Verification items for the finished model (mm, model axes). Face numbers are marked on the shaded views. A direction names the side the tool comes from. Round coordinates to 2 decimals unless told otherwise and drop trailing zeros. Order: outer loops, then holes, each group sorted by start corner. A loop starts at its lowest first (then second) coordinate and runs counter-clockwise, first axis right, second up. Notation, with made-up numbers: M 66.5,11 L 71.5,11 A16 ccw 71.5,18 Z; hole C 52.5,8 d11. An arc over 180 degrees is marked long. Return JSON: item names as keys, results as strings. Group by question number.
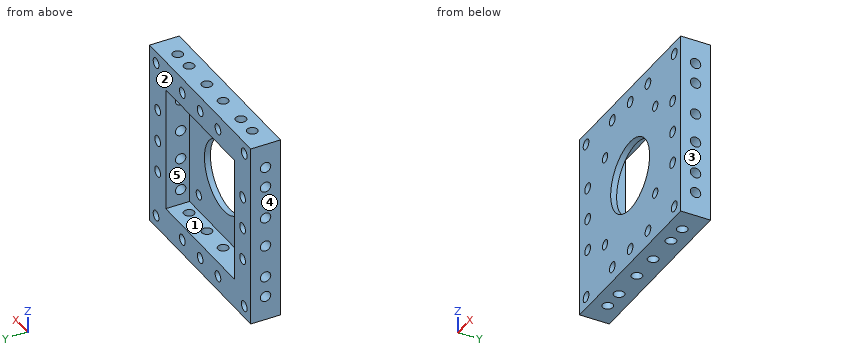
from build123d import *

# Parameters (mm, degrees)
SKETCH_1_W               = 42.4
SKETCH_1_H               = 42.4
EXTRUDE_1_DEPTH          = 2
SKETCH_2_W               = 62.4
SKETCH_2_H               = 62.4
SKETCH_2_W_2             = 42.4
SKETCH_2_H_2             = 42.4
EXTRUDE_2_DEPTH          = 10
CUT_EXTRUDE_1_REACH      = 4
SKETCH_5_R               = 1.6
SKETCH_5_R_2             = 12
CUT_EXTRUDE_START        = -10
SKETCH_7_R               = 1.75
CUT_EXTRUDE_3_DEPTH      = 10
PATTERN_CIRCULAR_2_COUNT = 4
CUT_EXTRUDE_2_REACH      = 12
SKETCH_6_R               = 1.75


with BuildPart() as part:
    # 草图1 → 凸台-拉伸1 (new body)
    with BuildSketch(Plane(origin=(0, 0, 0), x_dir=(1, 0, 0), z_dir=(0, 1, 0))):
        Rectangle(SKETCH_1_W, SKETCH_1_H)
    extrude(amount=EXTRUDE_1_DEPTH)

    # 草图2 → 凸台-拉伸2 (add)
    with BuildSketch(Plane(origin=(0, 0, 0), x_dir=(1, 0, 0), z_dir=(0, 1, 0))):
        Rectangle(SKETCH_2_W, SKETCH_2_H)
        Rectangle(SKETCH_2_W_2, SKETCH_2_H_2, mode=Mode.SUBTRACT)
    extrude(amount=EXTRUDE_2_DEPTH)

    # 草图5 → 切除-拉伸1 (cut, up to next)
    with BuildSketch(Plane(origin=(0, 2, 0), x_dir=(1, 0, 0), z_dir=(0, 1, 0)), mode=Mode.PRIVATE) as cut_extrude_1_sk1:
        with Locations((-15.5, 15.5)):
            Circle(SKETCH_5_R)
    cut_extrude_1_tool1 = extrude(cut_extrude_1_sk1.sketch, amount=-CUT_EXTRUDE_1_REACH, mode=Mode.PRIVATE) & part.part
    add(cut_extrude_1_tool1.solids().sort_by_distance((-15.5, 2, -15.5))[0], mode=Mode.SUBTRACT)
    # 草图5 → 切除-拉伸1 (cut, up to next)
    with BuildSketch(Plane(origin=(0, 2, 0), x_dir=(1, 0, 0), z_dir=(0, 1, 0)), mode=Mode.PRIVATE) as cut_extrude_1_sk2:
        with Locations((15.5, 15.5)):
            Circle(SKETCH_5_R)
    cut_extrude_1_tool2 = extrude(cut_extrude_1_sk2.sketch, amount=-CUT_EXTRUDE_1_REACH, mode=Mode.PRIVATE) & part.part
    add(cut_extrude_1_tool2.solids().sort_by_distance((15.5, 2, -15.5))[0], mode=Mode.SUBTRACT)
    # 草图5 → 切除-拉伸1 (cut, up to next)
    with BuildSketch(Plane(origin=(0, 2, 0), x_dir=(1, 0, 0), z_dir=(0, 1, 0)), mode=Mode.PRIVATE) as cut_extrude_1_sk3:
        with Locations((15.5, -15.5)):
            Circle(SKETCH_5_R)
    cut_extrude_1_tool3 = extrude(cut_extrude_1_sk3.sketch, amount=-CUT_EXTRUDE_1_REACH, mode=Mode.PRIVATE) & part.part
    add(cut_extrude_1_tool3.solids().sort_by_distance((15.5, 2, 15.5))[0], mode=Mode.SUBTRACT)
    # 草图5 → 切除-拉伸1 (cut, up to next)
    with BuildSketch(Plane(origin=(0, 2, 0), x_dir=(1, 0, 0), z_dir=(0, 1, 0)), mode=Mode.PRIVATE) as cut_extrude_1_sk4:
        with Locations((-15.5, -15.5)):
            Circle(SKETCH_5_R)
    cut_extrude_1_tool4 = extrude(cut_extrude_1_sk4.sketch, amount=-CUT_EXTRUDE_1_REACH, mode=Mode.PRIVATE) & part.part
    add(cut_extrude_1_tool4.solids().sort_by_distance((-15.5, 2, 15.5))[0], mode=Mode.SUBTRACT)
    # 草图5 → 切除-拉伸1 (cut, up to next)
    with BuildSketch(Plane(origin=(0, 2, 0), x_dir=(1, 0, 0), z_dir=(0, 1, 0)), mode=Mode.PRIVATE) as cut_extrude_1_sk5:
        Circle(SKETCH_5_R_2)
    cut_extrude_1_tool5 = extrude(cut_extrude_1_sk5.sketch, amount=-CUT_EXTRUDE_1_REACH, mode=Mode.PRIVATE) & part.part
    add(cut_extrude_1_tool5.solids().sort_by_distance((0, 2, 0))[0], mode=Mode.SUBTRACT)

    # 草图7 → 切除-拉伸3 (cut)
    with BuildSketch(Plane.ZY.offset(31.2).offset(CUT_EXTRUDE_START)):
        with Locations((-16, 5)):
            Circle(SKETCH_7_R)
        with Locations((16, 5)):
            Circle(SKETCH_7_R)
        with Locations((-23, 5)):
            Circle(SKETCH_7_R)
        with Locations((23, 5)):
            Circle(SKETCH_7_R)
        with Locations((-5, 5)):
            Circle(SKETCH_7_R)
        with Locations((5, 5)):
            Circle(SKETCH_7_R)
    cut_extrude_3 = extrude(amount=CUT_EXTRUDE_3_DEPTH, mode=Mode.SUBTRACT)

    # 阵列(圆周)2: 切除-拉伸3 ×4 about axis
    pattern_circular_2_axis = Axis((0, 0, 0), (0, 1, 0))
    for i in range(1, PATTERN_CIRCULAR_2_COUNT):
        add(cut_extrude_3.rotate(pattern_circular_2_axis, i * 360 / PATTERN_CIRCULAR_2_COUNT), mode=Mode.SUBTRACT)

    # 草图6 → 切除-拉伸2 (cut, up to next)
    with BuildSketch(Plane(origin=(0, 10, 0), x_dir=(1, 0, 0), z_dir=(0, 1, 0)), mode=Mode.PRIVATE) as cut_extrude_2_sk1:
        with Locations((-27.2, 27.2)):
            Circle(SKETCH_6_R)
    cut_extrude_2_tool1 = extrude(cut_extrude_2_sk1.sketch, amount=-CUT_EXTRUDE_2_REACH, mode=Mode.PRIVATE) & part.part
    add(cut_extrude_2_tool1.solids().sort_by_distance((-27.2, 10, -27.2))[0], mode=Mode.SUBTRACT)
    # 草图6 → 切除-拉伸2 (cut, up to next)
    with BuildSketch(Plane(origin=(0, 10, 0), x_dir=(1, 0, 0), z_dir=(0, 1, 0)), mode=Mode.PRIVATE) as cut_extrude_2_sk2:
        with Locations((-26.2, 11)):
            Circle(SKETCH_6_R)
    cut_extrude_2_tool2 = extrude(cut_extrude_2_sk2.sketch, amount=-CUT_EXTRUDE_2_REACH, mode=Mode.PRIVATE) & part.part
    add(cut_extrude_2_tool2.solids().sort_by_distance((-26.2, 10, -11))[0], mode=Mode.SUBTRACT)
    # 草图6 → 切除-拉伸2 (cut, up to next)
    with BuildSketch(Plane(origin=(0, 10, 0), x_dir=(1, 0, 0), z_dir=(0, 1, 0)), mode=Mode.PRIVATE) as cut_extrude_2_sk3:
        with Locations((-26.2, 0)):
            Circle(SKETCH_6_R)
    cut_extrude_2_tool3 = extrude(cut_extrude_2_sk3.sketch, amount=-CUT_EXTRUDE_2_REACH, mode=Mode.PRIVATE) & part.part
    add(cut_extrude_2_tool3.solids().sort_by_distance((-26.2, 10, 0))[0], mode=Mode.SUBTRACT)
    # 草图6 → 切除-拉伸2 (cut, up to next)
    with BuildSketch(Plane(origin=(0, 10, 0), x_dir=(1, 0, 0), z_dir=(0, 1, 0)), mode=Mode.PRIVATE) as cut_extrude_2_sk4:
        with Locations((-11, 26.2)):
            Circle(SKETCH_6_R)
    cut_extrude_2_tool4 = extrude(cut_extrude_2_sk4.sketch, amount=-CUT_EXTRUDE_2_REACH, mode=Mode.PRIVATE) & part.part
    add(cut_extrude_2_tool4.solids().sort_by_distance((-11, 10, -26.2))[0], mode=Mode.SUBTRACT)
    # 草图6 → 切除-拉伸2 (cut, up to next)
    with BuildSketch(Plane(origin=(0, 10, 0), x_dir=(1, 0, 0), z_dir=(0, 1, 0)), mode=Mode.PRIVATE) as cut_extrude_2_sk5:
        with Locations((0, 26.2)):
            Circle(SKETCH_6_R)
    cut_extrude_2_tool5 = extrude(cut_extrude_2_sk5.sketch, amount=-CUT_EXTRUDE_2_REACH, mode=Mode.PRIVATE) & part.part
    add(cut_extrude_2_tool5.solids().sort_by_distance((0, 10, -26.2))[0], mode=Mode.SUBTRACT)
    # 草图6 → 切除-拉伸2 (cut, up to next)
    with BuildSketch(Plane(origin=(0, 10, 0), x_dir=(1, 0, 0), z_dir=(0, 1, 0)), mode=Mode.PRIVATE) as cut_extrude_2_sk6:
        with Locations((11, 26.2)):
            Circle(SKETCH_6_R)
    cut_extrude_2_tool6 = extrude(cut_extrude_2_sk6.sketch, amount=-CUT_EXTRUDE_2_REACH, mode=Mode.PRIVATE) & part.part
    add(cut_extrude_2_tool6.solids().sort_by_distance((11, 10, -26.2))[0], mode=Mode.SUBTRACT)
    # 草图6 → 切除-拉伸2 (cut, up to next)
    with BuildSketch(Plane(origin=(0, 10, 0), x_dir=(1, 0, 0), z_dir=(0, 1, 0)), mode=Mode.PRIVATE) as cut_extrude_2_sk7:
        with Locations((27.2, 27.2)):
            Circle(SKETCH_6_R)
    cut_extrude_2_tool7 = extrude(cut_extrude_2_sk7.sketch, amount=-CUT_EXTRUDE_2_REACH, mode=Mode.PRIVATE) & part.part
    add(cut_extrude_2_tool7.solids().sort_by_distance((27.2, 10, -27.2))[0], mode=Mode.SUBTRACT)
    # 草图6 → 切除-拉伸2 (cut, up to next)
    with BuildSketch(Plane(origin=(0, 10, 0), x_dir=(1, 0, 0), z_dir=(0, 1, 0)), mode=Mode.PRIVATE) as cut_extrude_2_sk8:
        with Locations((26.2, 11)):
            Circle(SKETCH_6_R)
    cut_extrude_2_tool8 = extrude(cut_extrude_2_sk8.sketch, amount=-CUT_EXTRUDE_2_REACH, mode=Mode.PRIVATE) & part.part
    add(cut_extrude_2_tool8.solids().sort_by_distance((26.2, 10, -11))[0], mode=Mode.SUBTRACT)
    # 草图6 → 切除-拉伸2 (cut, up to next)
    with BuildSketch(Plane(origin=(0, 10, 0), x_dir=(1, 0, 0), z_dir=(0, 1, 0)), mode=Mode.PRIVATE) as cut_extrude_2_sk9:
        with Locations((26.2, 0)):
            Circle(SKETCH_6_R)
    cut_extrude_2_tool9 = extrude(cut_extrude_2_sk9.sketch, amount=-CUT_EXTRUDE_2_REACH, mode=Mode.PRIVATE) & part.part
    add(cut_extrude_2_tool9.solids().sort_by_distance((26.2, 10, 0))[0], mode=Mode.SUBTRACT)
    # 草图6 → 切除-拉伸2 (cut, up to next)
    with BuildSketch(Plane(origin=(0, 10, 0), x_dir=(1, 0, 0), z_dir=(0, 1, 0)), mode=Mode.PRIVATE) as cut_extrude_2_sk10:
        with Locations((26.2, -11)):
            Circle(SKETCH_6_R)
    cut_extrude_2_tool10 = extrude(cut_extrude_2_sk10.sketch, amount=-CUT_EXTRUDE_2_REACH, mode=Mode.PRIVATE) & part.part
    add(cut_extrude_2_tool10.solids().sort_by_distance((26.2, 10, 11))[0], mode=Mode.SUBTRACT)
    # 草图6 → 切除-拉伸2 (cut, up to next)
    with BuildSketch(Plane(origin=(0, 10, 0), x_dir=(1, 0, 0), z_dir=(0, 1, 0)), mode=Mode.PRIVATE) as cut_extrude_2_sk11:
        with Locations((27.2, -27.2)):
            Circle(SKETCH_6_R)
    cut_extrude_2_tool11 = extrude(cut_extrude_2_sk11.sketch, amount=-CUT_EXTRUDE_2_REACH, mode=Mode.PRIVATE) & part.part
    add(cut_extrude_2_tool11.solids().sort_by_distance((27.2, 10, 27.2))[0], mode=Mode.SUBTRACT)
    # 草图6 → 切除-拉伸2 (cut, up to next)
    with BuildSketch(Plane(origin=(0, 10, 0), x_dir=(1, 0, 0), z_dir=(0, 1, 0)), mode=Mode.PRIVATE) as cut_extrude_2_sk12:
        with Locations((11, -26.2)):
            Circle(SKETCH_6_R)
    cut_extrude_2_tool12 = extrude(cut_extrude_2_sk12.sketch, amount=-CUT_EXTRUDE_2_REACH, mode=Mode.PRIVATE) & part.part
    add(cut_extrude_2_tool12.solids().sort_by_distance((11, 10, 26.2))[0], mode=Mode.SUBTRACT)
    # 草图6 → 切除-拉伸2 (cut, up to next)
    with BuildSketch(Plane(origin=(0, 10, 0), x_dir=(1, 0, 0), z_dir=(0, 1, 0)), mode=Mode.PRIVATE) as cut_extrude_2_sk13:
        with Locations((0, -26.2)):
            Circle(SKETCH_6_R)
    cut_extrude_2_tool13 = extrude(cut_extrude_2_sk13.sketch, amount=-CUT_EXTRUDE_2_REACH, mode=Mode.PRIVATE) & part.part
    add(cut_extrude_2_tool13.solids().sort_by_distance((0, 10, 26.2))[0], mode=Mode.SUBTRACT)
    # 草图6 → 切除-拉伸2 (cut, up to next)
    with BuildSketch(Plane(origin=(0, 10, 0), x_dir=(1, 0, 0), z_dir=(0, 1, 0)), mode=Mode.PRIVATE) as cut_extrude_2_sk14:
        with Locations((-11, -26.2)):
            Circle(SKETCH_6_R)
    cut_extrude_2_tool14 = extrude(cut_extrude_2_sk14.sketch, amount=-CUT_EXTRUDE_2_REACH, mode=Mode.PRIVATE) & part.part
    add(cut_extrude_2_tool14.solids().sort_by_distance((-11, 10, 26.2))[0], mode=Mode.SUBTRACT)
    # 草图6 → 切除-拉伸2 (cut, up to next)
    with BuildSketch(Plane(origin=(0, 10, 0), x_dir=(1, 0, 0), z_dir=(0, 1, 0)), mode=Mode.PRIVATE) as cut_extrude_2_sk15:
        with Locations((-27.2, -27.2)):
            Circle(SKETCH_6_R)
    cut_extrude_2_tool15 = extrude(cut_extrude_2_sk15.sketch, amount=-CUT_EXTRUDE_2_REACH, mode=Mode.PRIVATE) & part.part
    add(cut_extrude_2_tool15.solids().sort_by_distance((-27.2, 10, 27.2))[0], mode=Mode.SUBTRACT)
    # 草图6 → 切除-拉伸2 (cut, up to next)
    with BuildSketch(Plane(origin=(0, 10, 0), x_dir=(1, 0, 0), z_dir=(0, 1, 0)), mode=Mode.PRIVATE) as cut_extrude_2_sk16:
        with Locations((-26.2, -11)):
            Circle(SKETCH_6_R)
    cut_extrude_2_tool16 = extrude(cut_extrude_2_sk16.sketch, amount=-CUT_EXTRUDE_2_REACH, mode=Mode.PRIVATE) & part.part
    add(cut_extrude_2_tool16.solids().sort_by_distance((-26.2, 10, 11))[0], mode=Mode.SUBTRACT)


solid = part.part
1. Cross-section at A-A (z = 0). Enter the section's corners in (x, y).
2. Go/stop test with flat-tipped pins: pin 1 (4 mm diameter, centred on y = 5, z = -16, fed in from -X); pin 2 (3 mm diameter, centred on x = -23, y = 5, fed in from -Z); pin 3 (5 mm diameter, centred on x = 15.5, z = 15.5, fed in from +Y); pin 4 (1 mm diameter, centred on y = 4.5, z = -23.5, fed in from -X). Record where each tip stops, or that it passes through.
3. Cross-section at D-D (z = 18.5). Enter the section's corners in (x, y).
4. Thickness scan on line 1 along Z through (x, y) = (15.5, 1.2); line 2 along X through (y, z) = (8.75, -2). Record the ranges inside material, lowest first. Write a range as from..to.
5. Cross-section at B-B (x = -26.2). Give the number of separate pieces and of enclosed holes in the cut face, plus the area to 3 significant figures.
6. Draft check along X on the marked faces 1, 2 and 3. Enter one of: +X half, -X half, draft (parallel to the pull), parting line (faces both ways), or undercut.
7. Access from +Z, -Z, +X, -X, +Y, -Y to the whole of each face (thin tool, end or side, straight path). Record for the marked faces 4 and 5.
Computed:
{
 "1": {"outline": "M -31.2,0 L -27.95,0 L -27.95,10 L -31.2,10 Z; M -24.45,0 L -12,0 L -12,2 L -21.2,2 L -21.2,10 L -24.45,10 Z; M 12,0 L 24.45,0 L 24.45,10 L 21.2,10 L 21.2,2 L 12,2 Z; M 27.95,0 L 31.2,0 L 31.2,10 L 27.95,10 Z"},
 "2": {"pin 1": "stops at x = -31.2", "pin 2": "stops at z = -21.2", "pin 3": "stops at y = 2", "pin 4": "stops at x = -21.2"},
 "3": {"outline": "M -31.2,0 L 31.2,0 L 31.2,10 L 21.2,10 L 21.2,2 L -21.2,2 L -21.2,10 L -31.2,10 Z"},
 "4": {"line 1": "z = -31.2..-17.1, -13.9..13.9, 17.1..31.2", "line 2": "x = -31.2..-21.2, 21.2..31.2"},
 "5": {"separate pieces": "6", "enclosed holes": "6", "area": "404 mm²"},
 "6": {"face 1": "undercut", "face 2": "draft", "face 3": "+X half"},
 "7": {"face 4": "+Z, -Z, -X, +Y, -Y", "face 5": "+Y"}
}
